The model under review builds one solid part; all positions refer to its coordinate system, in mm. Face numbers are marked on the shaded views. A direction names the side the tool comes from. Round coordinates to 2 decimals unless told otherwise and drop trailing zeros. Order: outer loops, then holes, each group sorted by start corner. A loop starts at its lowest first (then second) coordinate and runs counter-clockwise, first axis right, second up. Notation, with made-up numbers: M -18,2 L 40,2 A7 cw 40,7 Z; hole C -7,28.5 d10. An arc over 180 degrees is marked long. Answer as a JSON object with one key per item and string values. Group by question number.
1) Insertion check: pin 1 Ø4.5 at (x, y) = (58.74, 31.75) entering from -Z; pin 2 Ø1 at (x, y) = (32, 23.5) entering from +Z; pin 3 Ø8 at (y, z) = (23, 13) entering from +X; pin 4 Ø16.5 at (x, y) = (13, 34.5) entering from +Z. Each pin has a flat end and moves straight along its axis. Give the tip position at first contact, or say it passes through.
2) Consider section A-A, the plane y = 31.75. Count the separate pieces of the cut face and the enclosed holes in it, then the cut area to 3 significant figures.
3) Consider section C-C, the plane x = 8. Write out the cut boundary in (y, z) (1 decimal), then the cut area to 3 significant figures.
4) Consider section D-D, the plane x = 31.5. Write out the cut boundary in (y, z) (1 decimal), then the cut area to 3 significant figures.
5) The part is to be moulded in two halves that separate along X. For the marked faces 4, 5 and 6, say which applies: +X half, -X half, draft (parallel to the pull), parting line (faces both ways), or undercut.
6) To check wall thickness, follow line 1 (X direction, y = 56, z = 7.75); line 2 (X direction, y = 32, z = 5.25); line 3 (X direction, y = 31.75, z = 9.5). State the ranges of each line that lie inside material, in increasing order.
7) For the marked faces 1, 2 and 3, list the 3-axis set-ups (+Z, -Z, +X, -X, +Y, -Y) from which the entire face can be reached by the end or side of a thin tool; tool diameter is ignored.
```python
from build123d import *

# Parameters (mm, degrees)
SKETCH2_W                  = 63.5
SKETCH2_H                  = 63.5
SKETCH2_R                  = 5.1435
BOSS_EXTRUDE1_DEPTH        = 20.6375
SKETCH3_W                  = 31.75
SKETCH3_H                  = 15.875
CUT_EXTRUDE1_DEPTH         = 93.143401317
SKETCH4_W                  = 12.7
SKETCH4_H                  = 12.7
CUT_EXTRUDE2_DEPTH         = 93.143401317
SKETCH5_R                  = 12.7
CUT_EXTRUDE3_DEPTH         = 3.96875
SKETCH6_R                  = 12.7
SKETCH6_R_2                = 7.52475
CUT_EXTRUDE4_DEPTH         = 0.79375
FILLET1_R                  = 1.5875
F_10_CLEARANCE_HOLE1_D     = 5.6134
F_10_CLEARANCE_HOLE1_DEPTH = 25.4
F_10_CLEARANCE_HOLE1_TIP   = 1.686435499


with BuildPart() as part:
    # Sketch2 → Boss-Extrude1 (new body)
    with BuildSketch(Plane.XY):
        with Locations((31.75, 31.75)):
            Rectangle(SKETCH2_W, SKETCH2_H)
        with Locations((9.525, 31.75)):
            Circle(SKETCH2_R, mode=Mode.SUBTRACT)
    extrude(amount=BOSS_EXTRUDE1_DEPTH)

    # Sketch3 → Cut-Extrude1 (cut, through all)
    with BuildSketch(Plane.XZ):
        with Locations((34.925, 12.7)):
            Rectangle(SKETCH3_W, SKETCH3_H)
    extrude(amount=-CUT_EXTRUDE1_DEPTH, mode=Mode.SUBTRACT)

    # Sketch4 → Cut-Extrude2 (cut, through all)
    with BuildSketch(Plane.XZ):
        with Locations((57.15, 14.2875)):
            Rectangle(SKETCH4_W, SKETCH4_H)
    extrude(amount=-CUT_EXTRUDE2_DEPTH, mode=Mode.SUBTRACT)

    # Sketch5 → Cut-Extrude3 (cut)
    with BuildSketch(Plane.XY.offset(20.6375)):
        with Locations((9.525, 31.75)):
            Circle(SKETCH5_R)
    extrude(amount=-CUT_EXTRUDE3_DEPTH, mode=Mode.SUBTRACT)

    # Sketch6 → Cut-Extrude4 (cut)
    with BuildSketch(Plane.XY.offset(16.66875)):
        with Locations((9.525, 31.75)):
            Circle(SKETCH6_R)
        with Locations((9.525, 31.75)):
            Circle(SKETCH6_R_2, mode=Mode.SUBTRACT)
    extrude(amount=-CUT_EXTRUDE4_DEPTH, mode=Mode.SUBTRACT)

    # Fillet1
    fillet1_edges = [part.edges().sort_by_distance(p)[0] for p in [
        (19.05, 63.5, 12.7),
        (50.8, 63.5, 6.35),
        (19.05, 0, 12.7),
        (50.8, 0, 6.35),
        (63.5, 63.5, 3.96875),
        (63.5, 0, 3.96875),
        (31.75, 63.5, 0),
        (63.5, 31.75, 0),
        (19.05, 40.150260413, 18.25625),
        (19.05, 23.349739587, 18.25625),
        (31.75, 0, 0),
        (0, 40.150260413, 18.25625),
        (0, 23.349739587, 18.25625),
        (0, 31.75, 0),
        (19.05, 31.75, 15.875),
        (0, 31.75, 15.875),
        (0, 63.5, 10.31875),
        (0, 0, 10.31875),
    ]]
    fillet(fillet1_edges, radius=FILLET1_R)

    # #10 Clearance Hole1
    with Locations(Plane.XY.offset(20.6375)):
        with Locations((58.7375, 6.35), (58.7375, 31.75), (58.7375, 57.15)):
            Hole(F_10_CLEARANCE_HOLE1_D / 2, depth=F_10_CLEARANCE_HOLE1_DEPTH)
            with Locations((0, 0, -(F_10_CLEARANCE_HOLE1_DEPTH + F_10_CLEARANCE_HOLE1_TIP / 2))):  # 118° drill point
                Cone(0, F_10_CLEARANCE_HOLE1_D / 2, F_10_CLEARANCE_HOLE1_TIP, mode=Mode.SUBTRACT)


solid = part.part
```
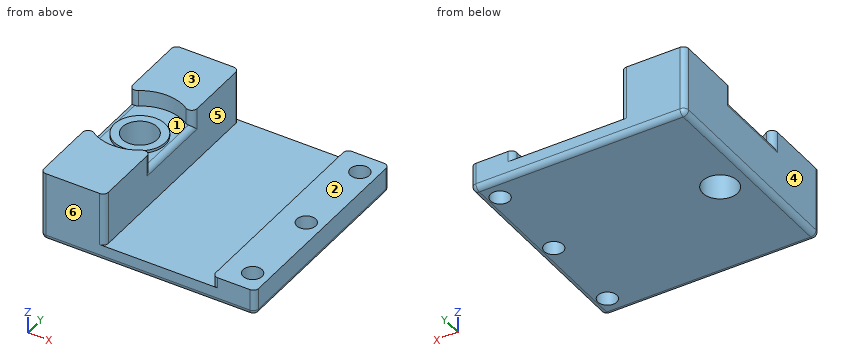
Results list:
{
 "1": {"pin 1": "through", "pin 2": "z = 4.76", "pin 3": "x = 19.05", "pin 4": "z = 16.67"},
 "2": {"separate pieces": "3", "enclosed holes": "0", "area": "348 mm^2"},
 "3": {"outline": "M 0,1.6 A1.6 ccw 1.6,0 L 26.8,0 L 26.8,16.7 L 24.4,16.7 L 24.4,15.9 L 19.1,15.9 L 19.1,20.6 L 0,20.6 Z; M 36.7,0 L 61.9,0 A1.6 ccw 63.5,1.6 L 63.5,20.6 L 44.4,20.6 L 44.4,15.9 L 39.1,15.9 L 39.1,16.7 L 36.7,16.7 Z", "area": "1,040 mm^2"},
 "4": {"outline": "M 0,1.6 A1.6 ccw 1.6,0 L 61.9,0 A1.6 ccw 63.5,1.6 L 63.5,4.8 L 0,4.8 Z", "area": "301 mm^2"},
 "5": {"face 4": "-X half", "face 5": "undercut", "face 6": "draft"},
 "6": {"line 1": "0 to 19.05, 50.8 to 56.18, 61.3 to 63.5", "line 2": "0 to 4.39, 14.66 to 19.05, 50.8 to 55.94, 61.53 to 63.5", "line 3": "0 to 4.38, 14.67 to 19.05"},
 "7": {"face 1": "+Z", "face 2": "+Z, +X, +Y, -Y", "face 3": "+Z, +X, -X, +Y, -Y"}
}
